from build123d import *

# Parameters (mm, degrees)
F0_R     = 2.25
F1_DEPTH = 3


with BuildPart() as f1:
    # F0 (on Front) → F1 (new body)
    with BuildSketch(Plane.XZ):
        Polygon((59.17797, 31.194587), (59.17797, 31.900588), (59.738858, 31.881615), (60.307068, 32.607616), (60.893968, 33.156025), (60.893968, 33.944442), (60.893968, 34.949179), (61.360855, 35.642351), (61.679476, 36.30662), (61.679476, 36.964568), (61.482426, 37.650985), (61.062581, 38.640238), (60.388171, 39.726486), (59.709248, 40.840028), (58.760794, 41.924554), (57.686546, 42.960874), (56.13193, 44.108019), (53.9429, 45.290024), (51.871779, 45.888075), (51.164123, 46.276766), (50.027608, 47.254788), (49.500446, 47.917502), (49.162385, 48.640302), (48.689091, 49.58215), (48.072106, 50.756746), (47.402845, 51.920425), (46.735066, 52.826829), (46.07114, 53.790702), (45.464824, 54.565684), (44.656431, 55.471539), (43.882285, 56.180216), (42.898628, 56.955005), (41.981423, 57.381575), (41.207883, 57.468069), (40.705001, 57.323706), (40.293103, 56.680384), (40.199735, 55.948148), (40.199735, 53.980475), (39.600259, 54.273897), (38.873113, 54.669222), (37.691645, 55.178945), (36.573572, 55.601232), (35.189915, 55.889827), (34.28163, 55.629085), (33.673137, 55.168423), (33.496248, 54.232587), (33.683778, 52.592809), (34.165904, 51.337972), (34.766386, 49.587351), (35.256976, 48.387687), (35.906764, 47.050612), (36.533276, 45.966415), (37.37989, 44.924222), (38.390851, 44.028023), (39.571477, 43.215491), (40.304705, 42.407678), (41.001196, 41.611003), (40.603713, 40.936851), (40.078084, 40.196856), (39.829461, 39.436208), (39.542939, 38.021807), (39.943556, 36.928817), (39.943556, 36.094203), (39.686826, 35.513923), (39.211509, 34.949179), (38.484942, 34.410313), (37.494795, 33.839713), (36.238837, 33.839713), (34.168248, 34.110547), (31.584672, 34.494312), (29.90189, 34.744845), (25.798248, 35.253315), (22.933811, 35.253315), (20.492591, 35.253315), (18.065328, 35.020179), (15.885449, 34.556809), (13.849761, 33.73976), (12.129347, 32.664482), (10.457839, 31.268078), (8.842911, 29.534917), (7.437296, 27.533482), (6.092134, 25.215313), (5.626353, 22.985314), (5.281105, 22.985314), (4.552305, 23.394156), (3.3653, 23.558287), (2.386902, 22.873478), (1.858065, 21.299662), (1.250321, 18.427405), (1.39535, 15.751299), (1.9034, 13.137148), (2.472708, 11.153989), (3.530675, 9.537014), (4.893567, 8.13821), (6.934674, 6.468246), (7.735685, 6.468246), (8.300671, 6.139061), (8.704288, 4.733078), (9.059932, 3.727228), (10.139112, 3.128539), (12.447312, 2.994476), (14.452639, 3.13662), (16.818212, 3.13662), (18.006043, 2.876388), (19.390354, 2.661495), (21.883129, 2.661495), (23.743564, 2.661495), (26.185988, 2.661495), (28.06579, 2.876388), (29.066299, 2.876388), (30.133199, 3.287267), (30.133199, 3.511565), (30.133199, 4.072266), (30.133199, 4.733231), (29.804504, 5.510292), (29.258075, 6.118042), (30.175305, 6.385948), (31.107011, 6.724561), (32.186629, 7.175799), (33.344732, 7.840062), (34.17739, 8.683063), (34.59618, 8.388327), (35.282453, 7.692138), (36.302242, 6.572426), (37.074772, 5.464323), (38.065363, 4.298558), (38.765096, 3.287267), (39.539397, 2.19271), (40.561764, 1.410144), (41.847485, 1.295176), (43.353376, 1.616231), (44.911167, 1.616231), (45.73869, 1.410144), (47.144735, 1.410144), (48.039055, 1.821825), (48.391114, 2.430058), (48.391114, 3.106444), (49.971162, 3.106444), (50.76906, 3.37499), (51.164123, 3.768711), (51.164123, 4.550725), (50.851106, 5.822739), (50.331727, 6.610573), (49.723235, 7.166963), (48.727288, 7.327425), (47.805995, 7.531474), (47.405892, 7.991314), (47.309159, 8.544259), (47.017634, 9.822114), (46.794978, 11.487763), (46.794978, 12.884877), (46.934963, 13.710026), (47.239665, 14.333159), (48.015684, 15.389006), (49.316895, 17.012446), (50.68293, 19.101975), (51.188018, 21.113079), (51.526973, 22.985314), (51.914252, 24.793496), (52.566426, 26.517666), (53.361181, 27.959348), (56.45878, 29.854865), (58.211347, 30.368955), align=None)
        with Locations((52.367389, 39.174978)):
            Circle(F0_R, mode=Mode.SUBTRACT)
    extrude(amount=F1_DEPTH)


solid = f1.part
Could you check a few things on this model? Use its own coordinates, in mm. A direction names the side the tool comes from. Give positions to 0.01 mm unless a question says otherwise; leave off trailing zeros. Order: outer loops, then holes, each group sorted by start corner. A loop starts at its lowest first (then second) coordinate and runs counter-clockwise, first axis right, second up.
1. For pin 1 (0.9 mm diameter, centred on y = -1.5, z = 36.5, fed in from -X); pin 2 (0.6 mm diameter, centred on y = -1, z = 4, fed in from +X); pin 3 (0.9 mm diameter, centred on x = 23, y = -2, fed in from +Z), each with a flat end and sliding along its axis, tell me the tip position at first contact or that it passes through.
Answers below:
pin 1: stops at x = 39.92
pin 2: stops at x = 51.16
pin 3: stops at z = 35.25
2. Which directions (+Z, -Z, +X, -X, +Y, -Y) give clear straight access to the entire face, cutting with the end or side of a thin tool? Please do faces 1 (the flat face through (35.577, -1.479, 47.729)), 2 (the flat face through (16, -1, 3.137)), 3 (the flat face through (47.165, -1.479, 9.174)), 4 (the flat face through (8.5, -1.48, 5.45)).
Answers below:
face 1: -X, +Y, -Y
face 2: -Z, +Y, -Y
face 3: +X, +Y, -Y
face 4: -Z, -X, +Y, -Y
3. Suppose I cut it at A-A (z = 20). Write out the boundary of the cut face in (x, y), plus the area to 3 significant figures.
Answers below:
outline: (1.58, -3) - (50.91, -3) - (50.91, 0) - (1.58, 0) - close
area: 148 mm2
4. I need wall thicknesses on L1, parallel to Z at x = 50.5, y = -0.25; L2, parallel to X at y = -1.55, z = 6; L3, parallel to X at y = -2, z = 38. Which ranges of each line are inside material? Lowest first, please.
Answers below:
L1: z = 3.28 to 6.36, 18.82 to 37.92, 40.43 to 46.85
L2: x = 8.34 to 29.36, 36.7 to 50.73
L3: x = 39.55 to 50.45, 54.29 to 61.33
5. Thinking about a two-plate mould opening in X: for faces 5 (the flat face through (39.69, -1.48, 38.74)), 6 (the flat face through (44, -1, 1.616)), 7 (the flat face through (46.795, -1, 12)), which applies, +X half, -X half, draft (parallel to the pull), parting line (faces both ways), or undercut?
Answers below:
face 5: -X half
face 6: undercut
face 7: +X half
